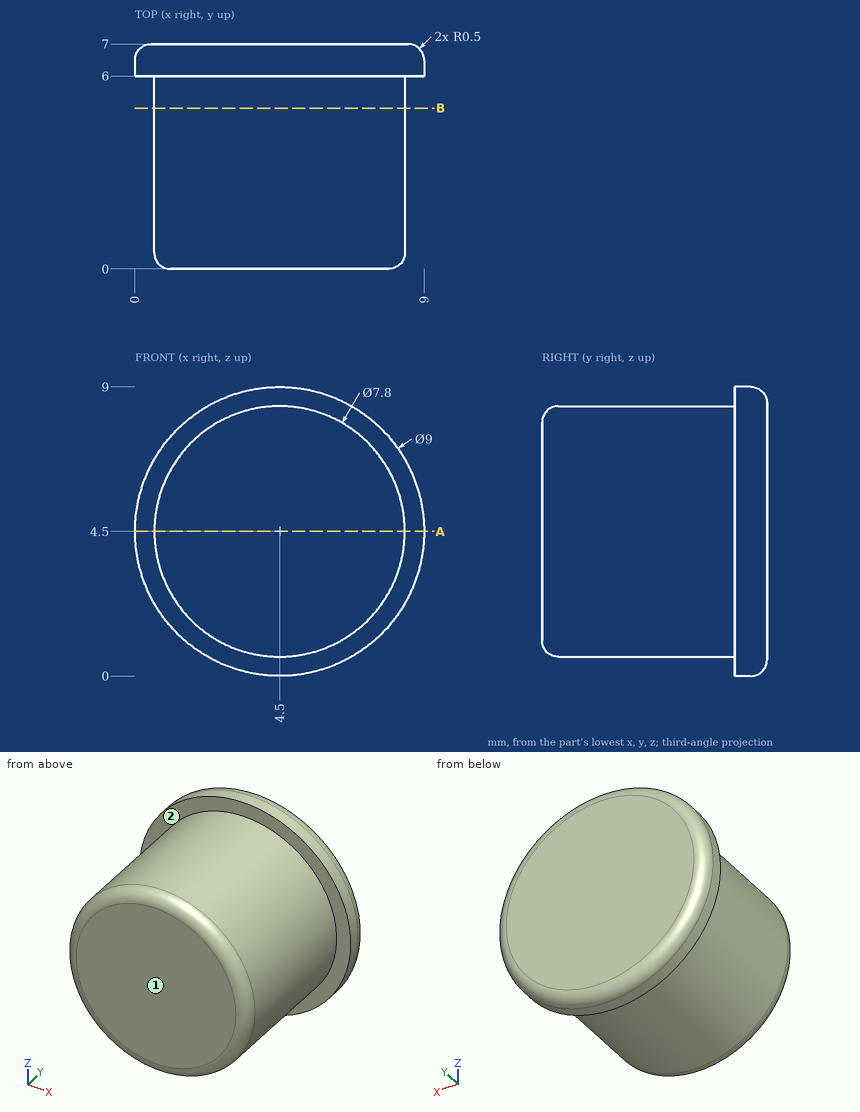
Study the drawing (mm; zero at the part's minimum x, y, z) and answer. A direction names the side the tool comes from. Give positions to 0.01 mm unless a question says otherwise; leave off trailing zeros. Order: outer loops, then holes, each group sorted by start corner. A loop starts at its lowest first (then second) coordinate and runs counter-clockwise, first axis right, second up. Notation, with made-up numbers: (82, 66.5) - (104, 66.5) arc R34 ccw to (104, 100.5) - close; hole circle Ø2 at (-24, 45.5). An arc over 180 degrees is marked (long way). Answer as CSV lines item,"result". Start each with the question number.
Q1. For the marked faces 1 and 2, determine the directions among +Z, -Z, +X, -X, +Y, -Y from which every point of the face is accessible in a straight line to the end or side of a thin tool.
Q2. Find the intervals of material crossed by L1, parallel to Z at x = 4.5, y = 3; L2, parallel to Y at x = 2, z = 1.75, in increasing order. Write a range as [from, to].
Q3. Given pin 1 Ø1 at (y, z) = (1, 5) entering from +X; pin 2 Ø2 at (x, y) = (7.5, 6) entering from -Z, each flat-ended and moving along its own axis, determine where each tip first touches the part or whether it passes through.
Q4. The part is cut by section B-B (y = 5). Write down the section's boundary in (x, z).
Q5. The part is cut by section A-A (z = 4.5). Write down the section's boundary in (x, y).
Check result:
1,face 1,"+Z, -Z, +X, -X, -Y"
1,face 2,"-Y"
2,L1,"z = [0.6, 8.4]"
2,L2,"y = [0.11, 7]"
3,pin 1,"stops at x = 8.4"
3,pin 2,"stops at z = 0.47"
4,outline,"circle Ø7.8 at (4.5, 4.5)"
5,outline,"(0, 6) - (0.6, 6) - (0.6, 0.5) arc R0.5 ccw to (1.1, 0) - (7.9, 0) arc R0.5 ccw to (8.4, 0.5) - (8.4, 6) - (9, 6) - (9, 6.5) arc R0.5 ccw to (8.5, 7) - (0.5, 7) arc R0.5 ccw to (0, 6.5) - close"
